Input: dimensioned drawing with shaded views. Units: mm. Origin: part minimum x, y, z. A direction names the side the tool comes from. Give positions to 0.01 mm unless a question says otherwise; leave off trailing zeros. Loops run counter-clockwise (first coordinate to the right, second up) from the corner with the lowest first, then second, coordinate; pieces in that order, holes last. Notation, with made-up numbers: M -26,34.25 L 15,34.25 A16 cw 15,42.25 Z; hole C -3,-10.5 d1. An arc over 180 degrees is marked long. Use CSV: the item, a comma, the result in double quotes. Start each with the question number.
Q1. Pull-direction query (X, two-part tool) for the marked faces 3, 4 and 5; classes: released by +X, released by -X, zero draft, split by the parting line, or undercut.
Q2. Section A-A, the plane z = 6.35. Output: boundary loops of the cut face in (x, y) (3 decimals).
Q3. Section C-C, the plane x = 14.5. Output: boundary loops of the cut face in (y, z), plus the area to 3 significant figures.
Q4. Pin query (flat end, axial travel): pin 1 (4 mm diameter, centred on x = 66.675, z = 6.35, fed in from +Y); pin 2 (2 mm diameter, centred on x = 71, z = 5.5, fed in from +Y). Return the tip coordinate at first contact, or that it passes through.
Q5. Reachability of the marked faces 1 and 2 from +Z, -Z, +X, -X, +Y, -Y: full face, straight path, thin tool, end or side. Return the list, or none.
Q6. Section B-B, the plane y = 113. Output: boundary loops of the cut face in (x, z), plus the area to 3 significant figures.
Q7. Material intervals for line 1 along X through (y, z) = (33, 5.5); line 2 along Z through (x, y) = (3, 120.65) (3 decimals); line 3 along Y through (x, z) = (86, 10), sorted ascending.
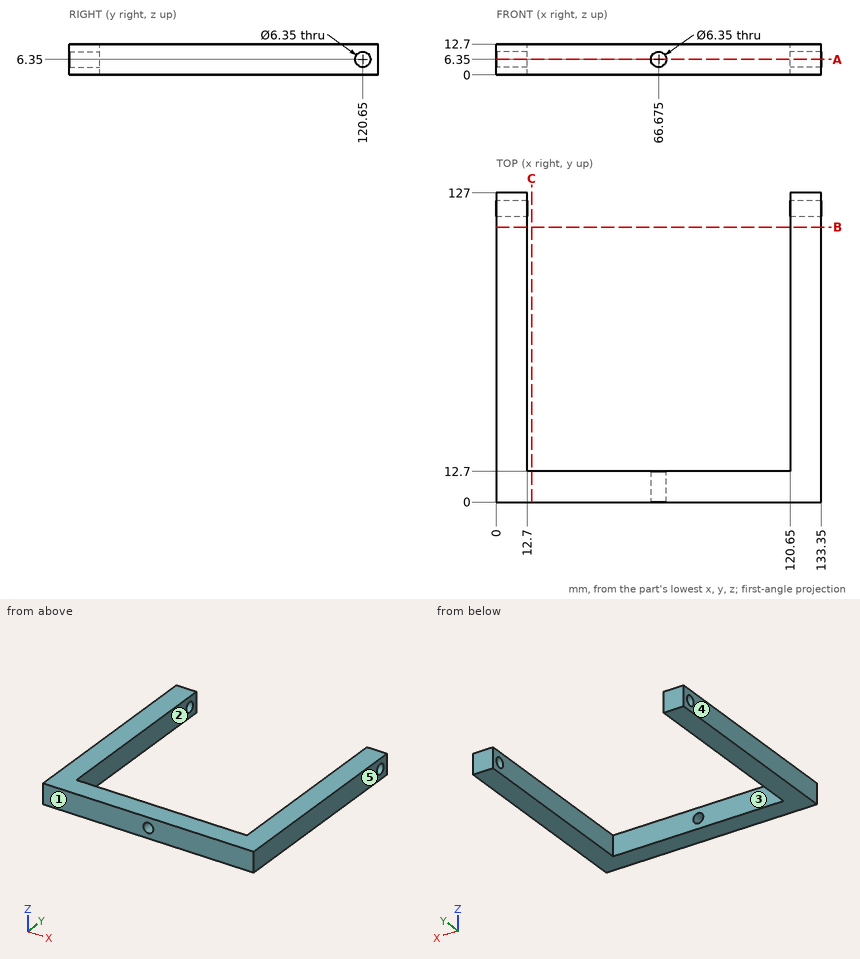
A:
1,face 3,"undercut"
1,face 4,"released by -X"
1,face 5,"released by +X"
2,outline,"M 0,0 L 63.5,0 L 63.5,12.7 L 12.7,12.7 L 12.7,117.475 L 0,117.475 Z; M 0,123.825 L 12.7,123.825 L 12.7,127 L 0,127 Z; M 69.85,0 L 133.35,0 L 133.35,117.475 L 120.65,117.475 L 120.65,12.7 L 69.85,12.7 Z; M 120.65,123.825 L 133.35,123.825 L 133.35,127 L 120.65,127 Z"
3,outline,"M 0,0 L 12.7,0 L 12.7,12.7 L 0,12.7 Z"
3,area,"161 mm^2"
4,pin 1,"through"
4,pin 2,"y = 12.7"
5,face 1,"+Z, -Z, +X, -X, -Y"
5,face 2,"+Z, -Z, +Y"
6,outline,"M 0,0 L 12.7,0 L 12.7,12.7 L 0,12.7 Z; M 120.65,0 L 133.35,0 L 133.35,12.7 L 120.65,12.7 Z"
6,area,"323 mm^2"
7,line 1,"0 to 12.7, 120.65 to 133.35"
7,line 2,"0 to 3.175, 9.525 to 12.7"
7,line 3,"0 to 12.7"
